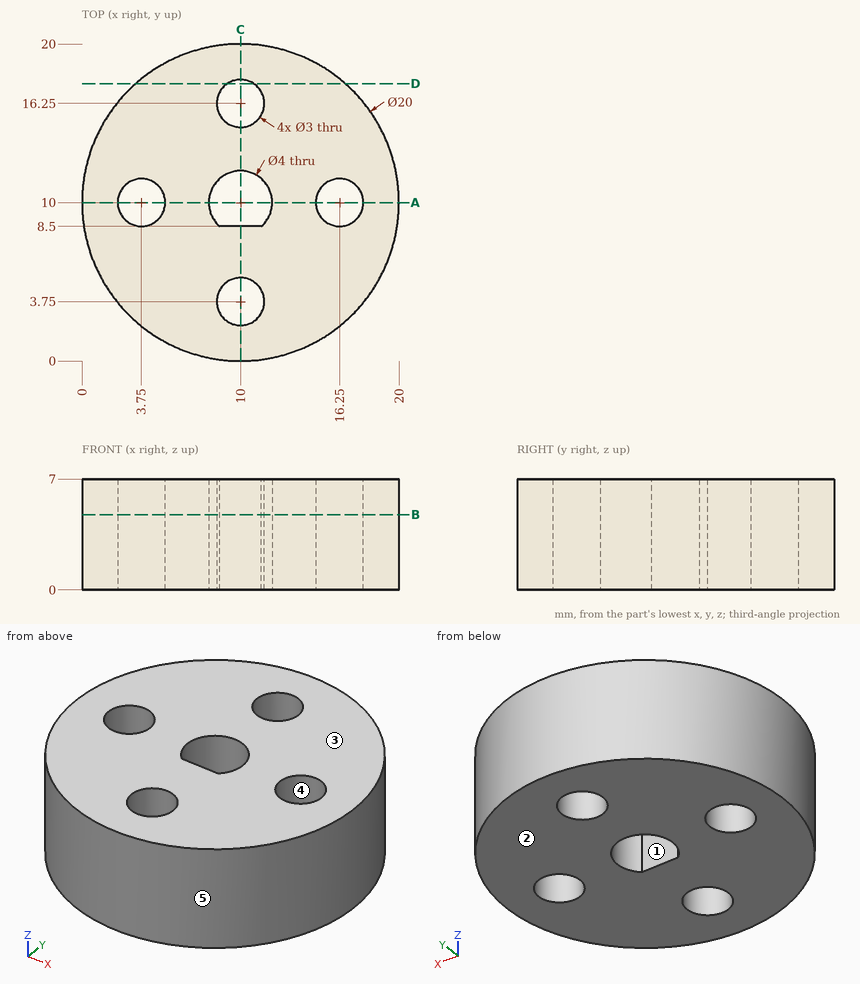
Design review of the part shown in the three views and the two pictorial views. Dimensions are in mm from the part's minimum x, y and z. A direction names the side the tool comes from. Round coordinates to 2 decimals unless told otherwise and drop trailing zeros. Loops run counter-clockwise (first coordinate to the right, second up) from the corner with the lowest first, then second, coordinate; pieces in that order, holes last. Notation, with made-up numbers: (85, 87.5) - (92, 87.5) arc R11 cw to (92, 91.5) - close; hole circle Ø9 at (55.5, 18.25). An arc over 180 degrees is marked (long way). Write each question's results on one line, items separated by ' | '. Start each with the question number.
Q1. Wall thickness on line 1 along Y through (x, z) = (10, 5.5); line 2 along Y through (x, z) = (16.25, 3.5); line 3 along Y through (x, z) = (8.25, 4.5): over which ranges is each line inside the solid? List them lowest first. Write a range as [from, to].
Q2. Tool access review of the marked faces 1 and 2: name each direction out of +Z, -Z, +X, -X, +Y, -Y from which nothing blocks a thin tool from reaching the whole face with its end or side.
Q3. Draft analysis for pull direction X (two halves, no side actions). For the marked faces 3, 4 and 5, state which applies: pulls with the +X half, pulls with the -X half, needs draft (parallel to the pull), parting line crosses it, or undercut.
Q4. Take a section at D-D on y = 17.5. Give the boundary of the cut face in (x, z), plus the area to 3 significant figures.
Q5. Take a section at B-B on z = 4.75. Give the boundary of the cut face in (x, y), plus the area to 3 significant figures.
Q6. Take a section at C-C on x = 10. Give the boundary of the cut face in (y, z).
Q7. Take a section at A-A on y = 10. Give the boundary of the cut face in (x, z), plus the area to 3 significant figures.
Data:
1) line 1: y = [0, 2.25], [5.25, 8.5], [12, 14.75], [17.75, 20] | line 2: y = [2.19, 8.5], [11.5, 17.81] | line 3: y = [0.15, 9.03], [10.97, 19.85]
2) face 1: +Z, -Z | face 2: -Z, +X, -X, +Y, -Y
3) face 3: needs draft | face 4: undercut | face 5: parting line crosses it
4) outline: (3.39, 0) - (9.17, 0) - (9.17, 7) - (3.39, 7) - close; (10.83, 0) - (16.61, 0) - (16.61, 7) - (10.83, 7) - close | area: 81.0 mm²
5) outline: circle Ø20 at (10, 10); hole circle Ø3 at (3.75, 10); hole circle Ø3 at (10, 3.75); hole circle Ø3 at (10, 16.25); hole (8.68, 8.5) - (11.32, 8.5) arc R2 ccw (long way) to start; hole circle Ø3 at (16.25, 10) | area: 274 mm²
6) outline: (0, 0) - (2.25, 0) - (2.25, 7) - (0, 7) - close; (5.25, 0) - (8.5, 0) - (8.5, 7) - (5.25, 7) - close; (12, 0) - (14.75, 0) - (14.75, 7) - (12, 7) - close; (17.75, 0) - (20, 0) - (20, 7) - (17.75, 7) - close
7) outline: (0, 0) - (2.25, 0) - (2.25, 7) - (0, 7) - close; (5.25, 0) - (8, 0) - (8, 7) - (5.25, 7) - close; (12, 0) - (14.75, 0) - (14.75, 7) - (12, 7) - close; (17.75, 0) - (20, 0) - (20, 7) - (17.75, 7) - close | area: 70.0 mm²
